```python
from build123d import *

# Parameters (mm, degrees)
F0_R     = 5
F1_DEPTH = 15
F2_R     = 2.25
F3_DEPTH = 5.5358573251


with BuildPart() as f1:
    # F0 (on Top) → F1 (new body)
    with BuildSketch(Plane.XY):
        with BuildLine():
            ThreePointArc((7, 10), (0, 17), (-7, 10))
            ThreePointArc((-7, 10), (0, 3), (7, 10))
        make_face()
        with Locations((0, 10)):
            Circle(F0_R, mode=Mode.SUBTRACT)
        with BuildLine():
            Line((-7, 10), (-7, 0))
            Line((-7, 0), (7, 0))
            Line((7, 0), (7, 10))
            ThreePointArc((7, 10), (0, 3), (-7, 10))
        make_face()
    extrude(amount=F1_DEPTH)

    # F2 (on face) → F3 (cut, through all)
    with BuildSketch(Plane.XZ):
        with Locations((0, 7.5)):
            Circle(F2_R)
    extrude(amount=-F3_DEPTH, mode=Mode.SUBTRACT)


solid = f1.part
```
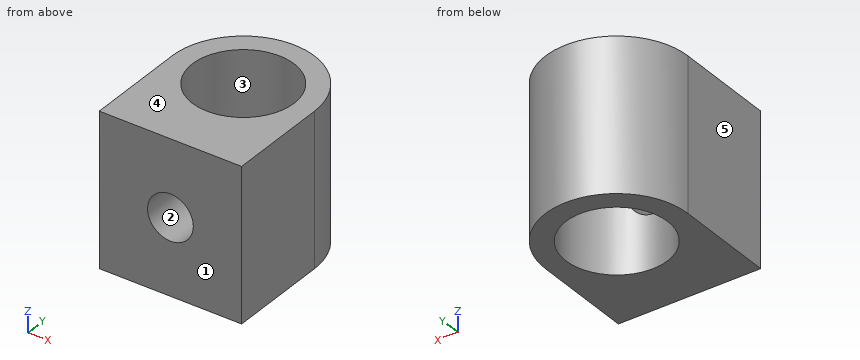
Here's how the part is built. I have some questions about the finished solid (model axes, mm). Face numbers are marked on the shaded views. A direction names the side the tool comes from. Coordinates: 2 decimals unless noted, no trailing zeros. Order: outer loops, then holes, each group sorted by start corner. A loop starts at its lowest first (then second) coordinate and runs counter-clockwise, first axis right, second up. Notation, with made-up numbers: (-1.5, 77) - (5.5, 77) arc R20 cw to (5.5, 111) - close; hole circle Ø10 at (14.25, 9). An arc over 180 degrees is marked (long way). One line per question, with ' | ' between items. Start each with the question number.
1. If we section it at C-C (y = 14.5): Write out the boundary of the cut face in (x, z), and give its area (3 significant figures).
2. If we mould it in two halves opening along X, with no side actions, what happens to the marked faces 3, 4 and 5? For each: released by +X, released by -X, zero draft, split by the parting line, or undercut.
3. If we section it at D-D (y = 2): Write out the boundary of the cut face in (x, z).
4. I'm going to push a flat-ended pin straight in: pin 1 Ø5 at (x, z) = (-5, 5) entering from -Y. Where does the tip first touch, or does it pass through?
5. If we section it at B-B (x = -4): Write out the boundary of the cut face in (y, z), and give its area (3 significant figures).
6. Please list where these lines run through material, in increasing order: line 1 along Y through (x, z) = (0, 3); line 2 along Z through (x, y) = (0, 4.4); line 3 along X through (y, z) = (2.75, 7.5). Write a range as [from, to].
7. Which directions (+Z, -Z, +X, -X, +Y, -Y) give clear straight access to the entire face, cutting with the end or side of a thin tool? Please do the marked faces 1 and 2.
8. If we section it at A-A (x = 0): Write out the boundary of the cut face in (y, z), and give its area (3 significant figures).
Model answer:
1) outline: (-5.36, 0) - (-2.18, 0) - (-2.18, 15) - (-5.36, 15) - close; (2.18, 0) - (5.36, 0) - (5.36, 15) - (2.18, 15) - close | area: 95.5 mm²
2) face 3: undercut | face 4: zero draft | face 5: released by -X
3) outline: (-7, 0) - (7, 0) - (7, 15) - (-7, 15) - close; hole circle Ø4.5 at (0, 7.5)
4) pin 1: stops at y = 0
5) outline: (0, 0) - (7, 0) - (7, 15) - (0, 15) - close; (13, 0) - (15.74, 0) - (15.74, 15) - (13, 15) - close | area: 146 mm²
6) line 1: y = [0, 5], [15, 17] | line 2: z = [0, 5.25], [9.75, 15] | line 3: x = [-7, -2.25], [2.25, 7]
7) face 1: +Z, -Z, +X, -X, -Y | face 2: -Y
8) outline: (0, 0) - (5, 0) - (5, 5.25) - (0, 5.25) - close; (0, 9.75) - (5, 9.75) - (5, 15) - (0, 15) - close; (15, 0) - (17, 0) - (17, 15) - (15, 15) - close | area: 82.5 mm²
